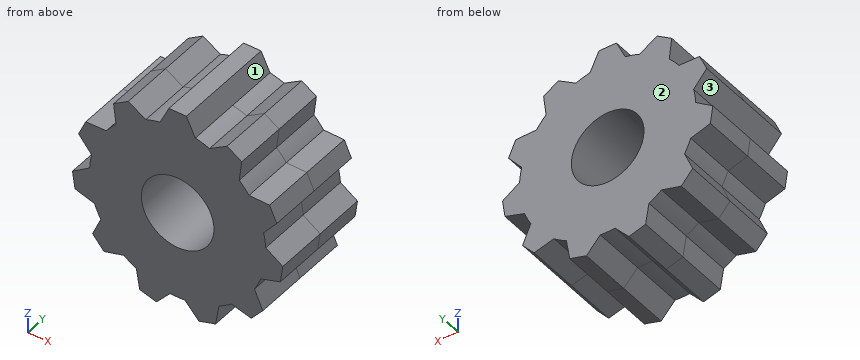
```python
from build123d import *

# Parameters (mm, degrees)
SKETCH1_R            = 3.5
BOSS_EXTRUDE1_DEPTH  = 5
SKETCH12_R           = 8.5
SKETCH12_R_2         = 3.5
BOSS_EXTRUDE6_DEPTH  = 5
BOSS_EXTRUDE9_DEPTH  = 5
CIRPATTERN2_COUNT    = 11
CUT_EXTRUDE1_START   = -10
SKETCH14_R           = 3.5
CUT_EXTRUDE1_DEPTH   = 10
SKETCH17_R           = 3.5
BOSS_EXTRUDE10_DEPTH = 5
BOSS_EXTRUDE11_DEPTH = 5


with BuildPart() as part:
    # Sketch1 → Boss-Extrude1 (new body)
    with BuildSketch(Plane(origin=(0, 0, 0), x_dir=(1, 0, 0), z_dir=(0, 1, 0))):
        with Locations(Location((0, 0, 0), (0, 0, 270))):
            Circle(SKETCH1_R)
    extrude(amount=BOSS_EXTRUDE1_DEPTH)

    # Sketch14 → Cut-Extrude1 (cut)
    with BuildSketch(Plane(origin=(0, 5, 0), x_dir=(1, 0, 0), z_dir=(0, 1, 0)).offset(CUT_EXTRUDE1_START)):
        with Locations(Location((0, 0, 0), (0, 0, 90))):
            Circle(SKETCH14_R)
    extrude(amount=CUT_EXTRUDE1_DEPTH, mode=Mode.SUBTRACT)


with BuildPart() as body_2:
    # Sketch12 → Boss-Extrude6 (new body)
    with BuildSketch(Plane(origin=(0, 5, 0), x_dir=(-1, 0, 0), z_dir=(0, -1, 0))):
        with Locations(Location((0, 0, 0), (0, 0, 90))):
            Circle(SKETCH12_R)
        with Locations(Location((0, 0, 0), (0, 0, 90))):
            Circle(SKETCH12_R_2, mode=Mode.SUBTRACT)
    extrude(amount=BOSS_EXTRUDE6_DEPTH)



with BuildPart() as body_3:
    # Sketch13 → Boss-Extrude9 (new body)
    with BuildSketch(Plane.XZ):
        with BuildLine():
            Line((1.7, 8.328265125), (0.84, 10.115181659))
            Line((0.84, 10.115181659), (-0.84, 10.115181659))
            Line((-0.84, 10.115181659), (-1.7, 8.328265125))
            ThreePointArc((-1.7, 8.328265125), (0, 8.5), (1.7, 8.328265125))
        make_face()
    extrude(amount=-BOSS_EXTRUDE9_DEPTH)


with BuildPart() as cirpattern2_1:
    # CirPattern2: pattern copy
    add(body_3.part.rotate(Axis((0, 0, 0), (0, 1, 0)), 1 * 360 / CIRPATTERN2_COUNT))


with BuildPart() as cirpattern2_2:
    # CirPattern2: pattern copy
    add(body_3.part.rotate(Axis((0, 0, 0), (0, 1, 0)), 2 * 360 / CIRPATTERN2_COUNT))


with BuildPart() as cirpattern2_3:
    # CirPattern2: pattern copy
    add(body_3.part.rotate(Axis((0, 0, 0), (0, 1, 0)), 3 * 360 / CIRPATTERN2_COUNT))


with BuildPart() as cirpattern2_4:
    # CirPattern2: pattern copy
    add(body_3.part.rotate(Axis((0, 0, 0), (0, 1, 0)), 4 * 360 / CIRPATTERN2_COUNT))


with BuildPart() as cirpattern2_5:
    # CirPattern2: pattern copy
    add(body_3.part.rotate(Axis((0, 0, 0), (0, 1, 0)), 5 * 360 / CIRPATTERN2_COUNT))


with BuildPart() as cirpattern2_6:
    # CirPattern2: pattern copy
    add(body_3.part.rotate(Axis((0, 0, 0), (0, 1, 0)), 6 * 360 / CIRPATTERN2_COUNT))


with BuildPart() as cirpattern2_7:
    # CirPattern2: pattern copy
    add(body_3.part.rotate(Axis((0, 0, 0), (0, 1, 0)), 7 * 360 / CIRPATTERN2_COUNT))


with BuildPart() as cirpattern2_8:
    # CirPattern2: pattern copy
    add(body_3.part.rotate(Axis((0, 0, 0), (0, 1, 0)), 8 * 360 / CIRPATTERN2_COUNT))


with BuildPart() as cirpattern2_9:
    # CirPattern2: pattern copy
    add(body_3.part.rotate(Axis((0, 0, 0), (0, 1, 0)), 9 * 360 / CIRPATTERN2_COUNT))


with BuildPart() as cirpattern2_10:
    # CirPattern2: pattern copy
    add(body_3.part.rotate(Axis((0, 0, 0), (0, 1, 0)), 10 * 360 / CIRPATTERN2_COUNT))


with BuildPart() as body_2_1:
    add(body_2.part)

    add(body_3.part)  # Boss-Extrude10 merges body 3

    add(cirpattern2_2.part)  # Boss-Extrude10 merges CirPattern2_2

    add(cirpattern2_3.part)  # Boss-Extrude10 merges CirPattern2_3

    add(cirpattern2_4.part)  # Boss-Extrude10 merges CirPattern2_4

    add(cirpattern2_5.part)  # Boss-Extrude10 merges CirPattern2_5

    add(cirpattern2_6.part)  # Boss-Extrude10 merges CirPattern2_6

    add(cirpattern2_7.part)  # Boss-Extrude10 merges CirPattern2_7

    add(cirpattern2_8.part)  # Boss-Extrude10 merges CirPattern2_8

    add(cirpattern2_9.part)  # Boss-Extrude10 merges CirPattern2_9

    add(cirpattern2_10.part)  # Boss-Extrude10 merges CirPattern2_10
    # Sketch17 → Boss-Extrude10 (add)
    with BuildSketch(Plane.XZ):
        with BuildLine():
            Line((5.180819576, -6.738628089), (7.094461217, -7.258864928))
            Line((7.094461217, -7.258864928), (8.19462725, -5.989205643))
            Line((8.19462725, -5.989205643), (7.407346071, -4.169079536))
            ThreePointArc((7.407346071, -4.169079536), (7.731871961, -3.531027611), (8.00156017, -2.867932156))
            Line((8.00156017, -2.867932156), (9.892679231, -2.270990453))
            Line((9.892679231, -2.270990453), (10.131768159, -0.608090431))
            Line((10.131768159, -0.608090431), (8.48543062, 0.497460747))
            ThreePointArc((8.48543062, 0.497460747), (8.413482256, 1.209676125), (8.281861946, 1.913311973))
            Line((8.281861946, 1.913311973), (9.550041487, 3.437907444))
            Line((9.550041487, 3.437907444), (8.852144265, 4.966089197))
            Line((8.852144265, 4.966089197), (6.869450902, 5.006060757))
            ThreePointArc((6.869450902, 5.006060757), (4.595446948, 7.150655029), (1.7, 8.328265125))
            Line((1.7, 8.328265125), (0.84, 10.115181659))
            Line((0.84, 10.115181659), (-0.84, 10.115181659))
            Line((-0.84, 10.115181659), (-1.7, 8.328265125))
            ThreePointArc((-1.7, 8.328265125), (-2.394726733, 8.155690276), (-3.07246906, 7.925271849))
            Line((-3.07246906, 7.925271849), (-4.762027113, 8.963570593))
            Line((-4.762027113, 8.963570593), (-6.175333049, 8.055294019))
            Line((-6.175333049, 8.055294019), (-5.932731071, 6.087093069))
            ThreePointArc((-5.932731071, 6.087093069), (-6.423871382, 5.566316239), (-6.869450902, 5.006060757))
            Line((-6.869450902, 5.006060757), (-8.852144265, 4.966089197))
            Line((-8.852144265, 4.966089197), (-9.550041487, 3.437907444))
            Line((-9.550041487, 3.437907444), (-8.281861946, 1.913311973))
            ThreePointArc((-8.281861946, 1.913311973), (-8.413482256, 1.209676125), (-8.48543062, 0.497460747))
            Line((-8.48543062, 0.497460747), (-10.131768159, -0.608090431))
            Line((-10.131768159, -0.608090431), (-9.892679231, -2.270990453))
            Line((-9.892679231, -2.270990453), (-8.00156017, -2.867932156))
            ThreePointArc((-8.00156017, -2.867932156), (-7.731871961, -3.531027611), (-7.407346071, -4.169079536))
            Line((-7.407346071, -4.169079536), (-8.19462725, -5.989205643))
            Line((-8.19462725, -5.989205643), (-7.094461217, -7.258864928))
            Line((-7.094461217, -7.258864928), (-5.180819576, -6.738628089))
            ThreePointArc((-5.180819576, -6.738628089), (-4.595446948, -7.150655029), (-3.977481483, -7.511966524))
            Line((-3.977481483, -7.511966524), (-3.65575009, -9.468790381))
            Line((-3.65575009, -9.468790381), (-2.043801894, -9.942101077))
            Line((-2.043801894, -9.942101077), (-0.715205373, -8.469857217))
            ThreePointArc((-0.715205373, -8.469857217), (0, -8.5), (0.715205373, -8.469857217))
            Line((0.715205373, -8.469857217), (2.043801894, -9.942101077))
            Line((2.043801894, -9.942101077), (3.65575009, -9.468790381))
            Line((3.65575009, -9.468790381), (3.977481483, -7.511966524))
            ThreePointArc((3.977481483, -7.511966524), (4.595446948, -7.150655029), (5.180819576, -6.738628089))
        make_face()
        with Locations(Location((0, 0, 0), (0, 0, 270))):
            Circle(SKETCH17_R, mode=Mode.SUBTRACT)
    extrude(amount=BOSS_EXTRUDE10_DEPTH)


    add(cirpattern2_1.part)  # Boss-Extrude11 merges CirPattern2_1
    # Sketch18 → Boss-Extrude11 (add)
    with BuildSketch(Plane.XZ):
        with BuildLine():
            Line((6.175333049, 8.055294019), (4.762027113, 8.963570593))
            Line((4.762027113, 8.963570593), (3.07246906, 7.925271849))
            ThreePointArc((3.07246906, 7.925271849), (4.595446948, 7.150655029), (5.932731071, 6.087093069))
            Line((5.932731071, 6.087093069), (6.175333049, 8.055294019))
        make_face()
    extrude(amount=BOSS_EXTRUDE11_DEPTH)


solid = body_2_1.part
```
Can you work these out from the model? Positions are in its coordinate system, mm. Face numbers are marked on the shaded views. Coordinates: 2 decimals unless noted, no trailing zeros. Loops run counter-clockwise (first coordinate to the right, second up) from the corner with the lowest first, then second, coordinate; pieces in that order, holes last. Notation, with made-up numbers: (-7, -15) -> (27, -15) arc R19 ccw to (27, 6) -> close; hole circle Ø3 at (-5.5, 66.5). An arc over 180 degrees is marked (long way). Put each result on its own line as item: value. Start each with the question number.
Q1. I'm going to push flat-ended pins straight in: P1, Ø4, axis at x = -4.5, y = -1.5, coming from the -Z side; P2, Ø3, axis at x = -3, y = -0.5, coming from the +Z side; P3, Ø5, axis at y = -3, z = 8, coming from the -X side. Where does each tip first touch, or does it pass through?
Q2. I want a section at B-B (z = 0.25). Write out the boundary of the cut face in (x, y).
Q3. I want a section at A-A (x = 0). Write out the boundary of the cut face in (y, z).
Q4. I want a section at D-D (x = -4.25). Write out the boundary of the cut face in (y, z).
Q5. Thinking about a two-plate mould opening in X: for the marked faces 1, 2 and 3, which applies, pulls with the +X half, pulls with the -X half, needs draft (parallel to the pull), parting line crosses it, or undercut?
Q6. I want a section at C-C (z = 5.75). Write out the boundary of the cut face in (x, y).
Q7. If I drill on line 1 (X direction, y = 0.25, z = 8.75); line 2 (X direction, y = -1, z = 0); line 3 (Z direction, x = 0.75, y = -3.75), over which ranges is the centre line in solid material (lowest first)? Write a range as [from, to].
Taken from the geometry:
1. P1: stops at z = -9.81
1. P2: stops at z = 8.8
1. P3: stops at x = -6.48
2. outline: (-8.85, -5) -> (-3.49, -5) -> (-3.49, 5) -> (-8.85, 5) -> close; (3.49, -5) -> (8.85, -5) -> (8.85, 5) -> (3.49, 5) -> close
3. outline: (-5, -8.5) -> (5, -8.5) -> (5, -3.5) -> (-5, -3.5) -> close; (-5, 3.5) -> (5, 3.5) -> (5, 10.12) -> (-5, 10.12) -> close
4. outline: (-5, -7.36) -> (5, -7.36) -> (5, 8.65) -> (-5, 8.65) -> close
5. face 1: undercut
5. face 2: needs draft
5. face 3: pulls with the -X half
6. outline: (-6.26, -5) -> (6.26, -5) -> (6.26, 5) -> (-6.26, 5) -> close
7. line 1: x = [-5.09, -4.41], [-1.5, 1.5], [4.41, 5.09]
7. line 2: x = [-9.23, -3.5], [3.5, 9.23]
7. line 3: z = [-8.51, -3.42], [3.42, 10.12]
